```python
from build123d import *

# Parameters (mm, degrees)
F1_DEPTH    = 6
F2_DEPTH    = 10
F3_T1_DEPTH = 82.1983443527


# Not quite as in the source:
# - a fillet or chamfer that OpenCascade refuses, or shapes differently, is made with other operations: its cross-section is extruded or revolved along the edge and cut away or added


with BuildPart() as f1:
    # F0 (on Front) → F1 (new body)
    with BuildSketch(Plane.XZ):
        with BuildLine():
            Line((10.5583761781, 15.9778866861), (-19.4416238219, 15.9778866861))
            Line((-19.4416238219, 15.9778866861), (-19.4416238219, 9.2778866861))
            Line((-19.4416238219, 9.2778866861), (-6.2031285903, 9.2778866861))
            ThreePointArc((-6.2031285903, 9.2778866861), (-8.2160972802, 15.0771908879), (-2.5916238219, 12.6176644117))
            ThreePointArc((-2.5916238219, 12.6176644117), (-3.4820973456, 10.3431909533), (-5.6801190534, 9.2778866861))
            Line((-5.6801190534, 9.2778866861), (10.5583761781, 9.2778866861))
            Line((10.5583761781, 9.2778866861), (10.5583761781, 15.9778866861))
        make_face()
        with BuildLine():
            ThreePointArc((-2.5916238219, 12.6176644117), (-8.2160972802, 15.0771908879), (-6.2031285903, 9.2778866861))
            Line((-6.2031285903, 9.2778866861), (-5.6801190534, 9.2778866861))
            ThreePointArc((-5.6801190534, 9.2778866861), (-3.4820973456, 10.3431909533), (-2.5916238219, 12.6176644117))
        make_face()
    extrude(amount=F1_DEPTH)

    # F0 (on Front) → F2 (join)
    with BuildSketch(Plane.XZ):
        with BuildLine():
            ThreePointArc((-2.5916238219, 12.6176644117), (-8.2160972802, 15.0771908879), (-6.2031285903, 9.2778866861))
            Line((-6.2031285903, 9.2778866861), (-5.6801190534, 9.2778866861))
            ThreePointArc((-5.6801190534, 9.2778866861), (-3.4820973456, 10.3431909533), (-2.5916238219, 12.6176644117))
        make_face()
    extrude(amount=-F2_DEPTH)

    # F3: fillet of radius 22 on 2 edges, made by hand

    # F3_s2 → F3_t1 (cut)
    with BuildSketch(Plane.XY.offset(-28.4712854902)):
        with BuildLine():
            ThreePointArc((-19.4416238219, 0), (-12.4659933559, -4.4450483003), (-4.3419549513, -6))
            Line((-4.3419549513, -6), (-19.4416238219, -6))
            Line((-19.4416238219, -6), (-19.4416238219, 0))
        make_face()
        with BuildLine():
            ThreePointArc((10.5583761781, 0), (3.5827457122, -4.4450483003), (-4.5412926924, -6))
            Line((-4.5412926924, -6), (10.5583761781, -6))
            Line((10.5583761781, -6), (10.5583761781, 0))
        make_face()
    extrude(amount=F3_T1_DEPTH, mode=Mode.SUBTRACT)


solid = f1.part
```
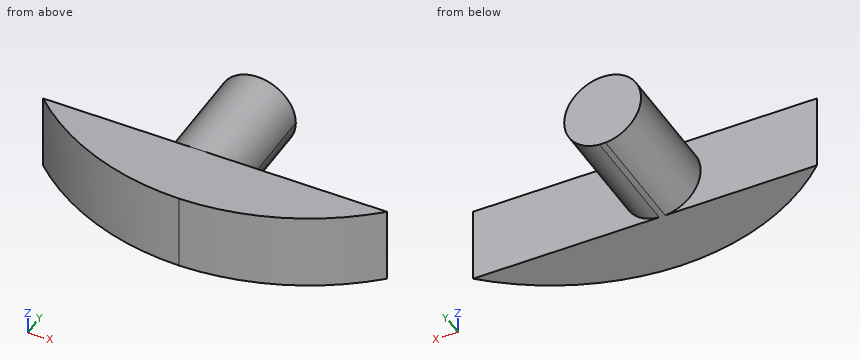
Geometry: final body of the model. Coordinates: model frame, mm. Coordinates: 2 decimals unless noted, no trailing zeros. Order: outer loops, then holes, each group sorted by start corner. A loop starts at its lowest first (then second) coordinate and runs counter-clockwise, first axis right, second up. Notation, with made-up numbers: (18, 71.25) -> (73, 71.25) arc R15 cw to (73, 99.25) -> close; hole circle Ø8 at (78, 12.5). An arc over 180 degrees is marked (long way). Answer in a Markdown table with one row per item.
Item 1: Section A-A on z = 13.75. Output: boundary loops of the cut face in (x, y), plus the area to 3 significant figures.
Return value:
| item | result |
|---|---|
| outline | (-19.44, 0) arc R22 ccw to (-4.44, -6) arc R22 ccw to (10.56, 0) -> (-2.79, 0) -> (-2.79, 10) -> (-9.09, 10) -> (-9.09, 0) -> close |
| area | 186 mm² |
Item 2: Section B-B on x = 1.5. Output: boundary loops of the cut face in (y, z), plus the area to 3 significant figures.
Return value:
| item | result |
|---|---|
| outline | (-5.15, 9.28) -> (0, 9.28) -> (0, 15.98) -> (-5.15, 15.98) -> close |
| area | 34.5 mm² |
Item 3: Ray query, L1, parallel to X at y = 8.5, z = 13.5; L2, parallel to Y at x = -5.5, z = 12.5; L3, parallel to Y at x = -13, z = 13.5. Return the intervals inside material, ascending.
Return value:
| item | result |
|---|---|
| L1 | x = -9.17 to -2.71 |
| L2 | y = -5.97 to 10 |
| L3 | y = -4.22 to 0 |
Item 4: Section C-C on z = 10. Output: boundary loops of the cut face in (x, y), plus the area to 3 significant figures.
Return value:
| item | result |
|---|---|
| outline | (-19.44, 0) arc R22 ccw to (-4.44, -6) arc R22 ccw to (10.56, 0) -> (-3.85, 0) -> (-3.85, 10) -> (-8.03, 10) -> (-8.03, 0) -> close |
| area | 165 mm² |
Item 5: Contact query for flat-ended pins moving along their axis: P1, Ø3, axis at x = -12.5, z = 10, coming from the +Y side; P2, Ø4, axis at y = -1, z = 14, coming from the -X side; P3, Ø1.5, axis at y = 5, z = 15, coming from the +X side. Output: stop coordinate, or through.
Return value:
| item | result |
|---|---|
| P1 | stops at y = 0 |
| P2 | stops at x = -19.44 |
| P3 | stops at x = -3.02 |
Item 6: Section D-D on y = 2. Output: boundary loops of the cut face in (x, z), plus the area to 3 significant figures.
Return value:
| item | result |
|---|---|
| outline | (-6.2, 9.28) -> (-5.68, 9.28) arc R3.35 ccw (long way) to start |
| area | 35.3 mm² |
